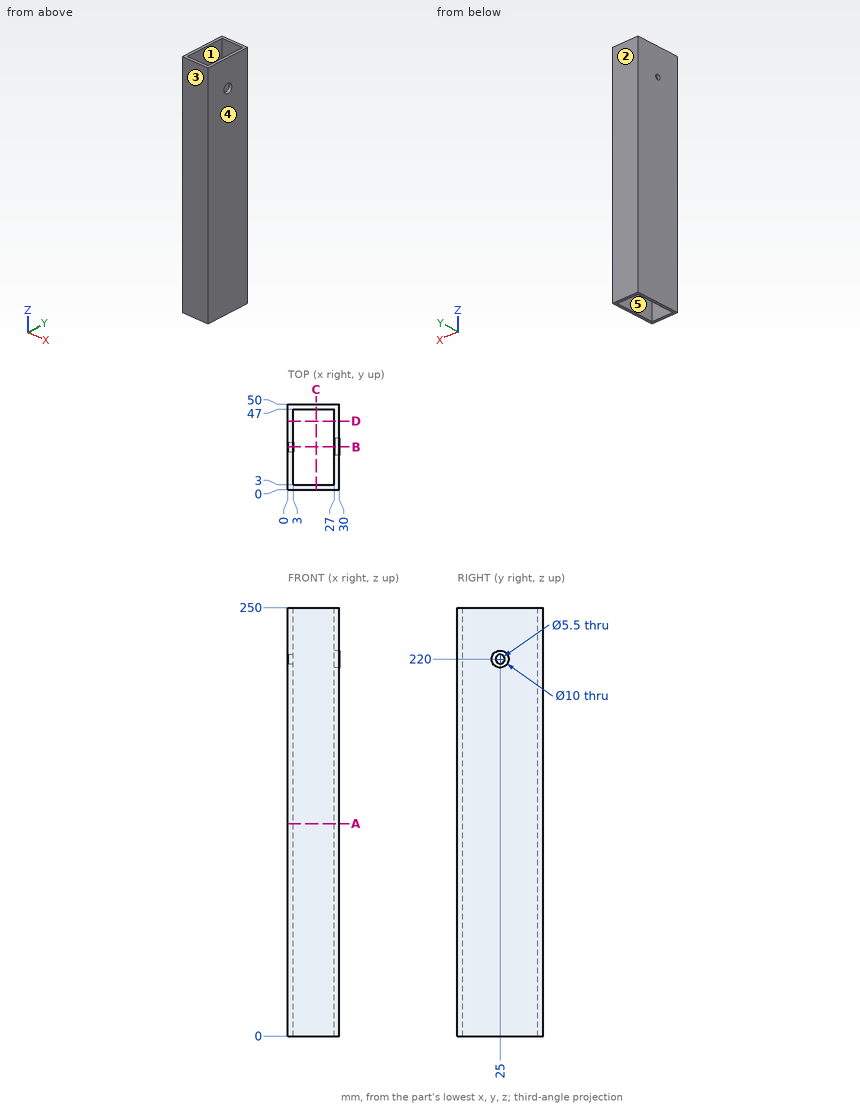
Can you work these out from the drawing? Everything is in mm from the part's minimum corner. A direction names the side the tool comes from. Round coordinates to 2 decimals unless told otherwise and drop trailing zeros. Loops run counter-clockwise (first coordinate to the right, second up) from the corner with the lowest first, then second, coordinate; pieces in that order, holes last. Notation, with made-up numbers: M 53.5,-23.75 L 75.5,-23.75 A25 cw 75.5,7.25 Z; hole C 12.5,-34.5 d3. An arc over 180 degrees is marked long. Answer in a Markdown table with one row per item.
1. Please list where these lines run through material, in increasing order: line 1 (Y direction, x = 2.05, z = 220); line 2 (Y direction, x = 23.25, z = 33); line 3 (X direction, y = 10.5, z = 30). Write a range as from..to.
Established:
| item | result |
|---|---|
| line 1 | 0..22.25, 27.75..50 |
| line 2 | 0..3, 47..50 |
| line 3 | 0..3, 27..30 |
2. If we section it at A-A, the plane z = 124: Please give me the cut outline in (x, y), plus the area to 3 significant figures.
Established:
| item | result |
|---|---|
| outline | M 0,0 L 30,0 L 30,50 L 0,50 Z; hole M 3,3 L 27,3 L 27,47 L 3,47 Z |
| area | 444 mm² |
3. If we section it at D-D, the plane y = 40: Please give me the cut outline in (x, z), plus the area to 3 significant figures.
Established:
| item | result |
|---|---|
| outline | M 0,0 L 3,0 L 3,250 L 0,250 Z; M 27,0 L 30,0 L 30,250 L 27,250 Z |
| area | 1,500 mm² |
4. If we section it at C-C, the plane x = 16.5: Please give me the cut outline in (y, z), plus the area to 3 significant figures.
Established:
| item | result |
|---|---|
| outline | M 0,0 L 3,0 L 3,250 L 0,250 Z; M 47,0 L 50,0 L 50,250 L 47,250 Z |
| area | 1,500 mm² |
5. If we section it at B-B, the plane y = 25: Please give me the cut outline in (x, z), plus the area to 3 significant figures.
Established:
| item | result |
|---|---|
| outline | M 0,0 L 3,0 L 3,217.25 L 0,217.25 Z; M 0,222.75 L 3,222.75 L 3,250 L 0,250 Z; M 27,0 L 30,0 L 30,215 L 27,215 Z; M 27,225 L 30,225 L 30,250 L 27,250 Z |
| area | 1,450 mm² |
6. Thinking about a two-plate mould opening in Y: for the marked faces 1, 2 and 3, which applies, pulls with the +Y half, pulls with the -Y half, needs draft (parallel to the pull), parting line crosses it, or undercut?
Established:
| item | result |
|---|---|
| face 1 | undercut |
| face 2 | pulls with the +Y half |
| face 3 | pulls with the -Y half |
7. On a 3-axis mill with a long thin cutter (end or side, diameter ignored), from which of +Z, -Z, +X, -X, +Y, -Y can I reach the whole of each face in a straight line? I mean the marked faces 4 and 5. Say none if no direction works.
Established:
| item | result |
|---|---|
| face 4 | +Z, -Z, +X, +Y, -Y |
| face 5 | +Z, -Z |
